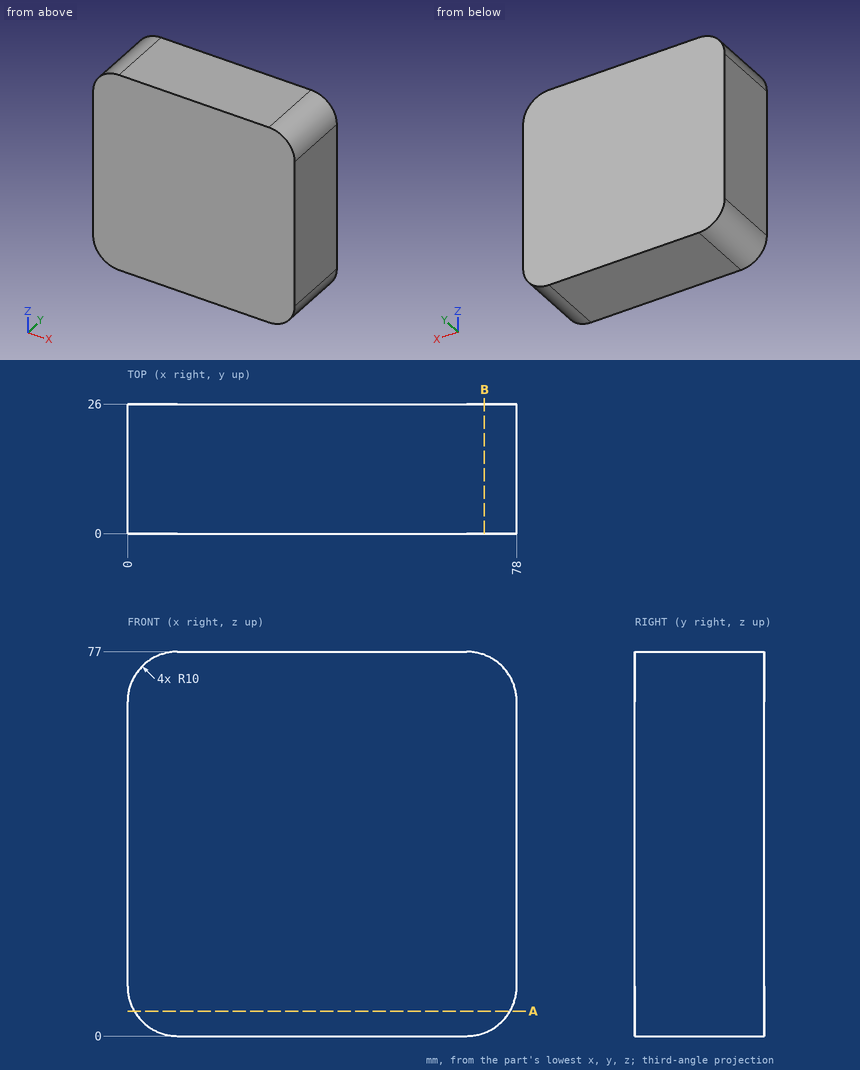
Geometry check sheet. Reference: drawing and pictorial views, mm from the part's lowest x, y, z. Round coordinates to 2 decimals unless told otherwise and drop trailing zeros. Loops run counter-clockwise (first coordinate to the right, second up) from the corner with the lowest first, then second, coordinate; pieces in that order, holes last.
1. Sectioned sample at A-A on z = 5. Record the boundary of the cut face in (x, y).
2. Scan lines: probe 1 along X at (y, z) = (12.5, 67.5); probe 2 along X at (y, z) = (7, 73.5); probe 3 along Z at (x, y) = (9.5, 12.5). Record each from-to range of solid material in increasing order.
3. Sectioned sample at B-B on x = 71.5. Record the boundary of the cut face in (y, z).
Recorded:
1. outline: (1.34, 0) - (76.66, 0) - (76.66, 26) - (1.34, 26) - close
2. probe 1: x = 0.01 to 77.99
2. probe 2: x = 2.4 to 75.6
2. probe 3: z = 0.01 to 76.99
3. outline: (0, 0.63) - (26, 0.63) - (26, 76.37) - (0, 76.37) - close
